from build123d import *
from build123d.topology import SkipClean

# Parameters (mm, degrees)
SKETCH_1_W          = 15
SKETCH_1_H          = 32.4
EXTRUDE_1_DEPTH     = 2.2
SKETCH_1_3_R        = 6.25
SKETCH_1_3_R_2      = 3
CUT_EXTRUDE_1_DEPTH = 36.771497033
SKETCH_2_W          = 15
SKETCH_2_H          = 32.4
EXTRUDE_2_DEPTH     = 4
SKETCH_3_R          = 0.8
CUT_EXTRUDE_2_DEPTH = 3
SKETCH_4_R          = 1
CUT_EXTRUDE_3_DEPTH = 36.927148509
SKETCH_4_3_R        = 1.5
SKETCH_4_3_R_2      = 1
CUT_EXTRUDE_4_DEPTH = 1.2


with BuildPart() as part:
    # Sketch 1 → Extrude 1 (new body)
    with BuildSketch(Plane(origin=(0, 0, 0), x_dir=(1, 0, 0), z_dir=(0, 1, 0))):
        with Locations((7.5, -16.2)):
            Rectangle(SKETCH_1_W, SKETCH_1_H)
    extrude(amount=EXTRUDE_1_DEPTH)

    # Sketch 1_3 → Cut-Extrude 1 (cut, through all)
    with BuildSketch(Plane(origin=(0, 0, 0), x_dir=(1, 0, 0), z_dir=(0, 1, 0))):
        with Locations((7.5, -21.35)):
            Circle(SKETCH_1_3_R)
        with Locations((7.5, -15.6)):
            Circle(SKETCH_1_3_R_2)
    extrude(amount=CUT_EXTRUDE_1_DEPTH, mode=Mode.SUBTRACT)

    # Sketch 2 → Extrude 2 (add)
    with SkipClean():  # the faces are left unmerged after this step: merging them gives an invalid solid
        with BuildSketch(Plane(origin=(0, 2.2, 0), x_dir=(1, 0, 0), z_dir=(0, 1, 0))):
            with Locations((7.5, -16.2)):
                Rectangle(SKETCH_2_W, SKETCH_2_H)
            with BuildLine():
                Line((1.3, -4.5), (13.7, -4.5))
                Line((13.7, -4.5), (13.7, -20.561013308))
                ThreePointArc((13.7, -20.561013308), (13.75, -21.35), (13.7, -22.138986692))
                Line((13.7, -22.138986692), (13.7, -27.9))
                Line((13.7, -27.9), (1.3, -27.9))
                Line((1.3, -27.9), (1.3, -22.138986692))
                ThreePointArc((1.3, -22.138986692), (1.25, -21.35), (1.3, -20.561013308))
                Line((1.3, -20.561013308), (1.3, -4.5))
            make_face(mode=Mode.SUBTRACT)
        extrude(amount=EXTRUDE_2_DEPTH)

    # Sketch 3 → Cut-Extrude 2 (cut)
    with SkipClean():  # the faces are left unmerged after this step: merging them gives an invalid solid
        with BuildSketch(Plane(origin=(0, 6.2, 0), x_dir=(1, 0, 0), z_dir=(0, 1, 0))):
            with Locations(Location((7.5, -30.3, 0), (0, 0, 180))):
                Circle(SKETCH_3_R)
            with Locations(Location((7.5, -2.1, 0), (0, 0, 180))):
                Circle(SKETCH_3_R)
        extrude(amount=-CUT_EXTRUDE_2_DEPTH, mode=Mode.SUBTRACT)

    # Sketch 4 → Cut-Extrude 3 (cut, through all)
    with SkipClean():  # the faces are left unmerged after this step: merging them gives an invalid solid
        with BuildSketch(Plane(origin=(0, 2.2, 0), x_dir=(1, 0, 0), z_dir=(0, 1, 0))):
            with Locations(Location((11.5, -11.35, 0), (0, 0, 270))):
                Circle(SKETCH_4_R)
            with Locations(Location((3.5, -11.35, 0), (0, 0, 270))):
                Circle(SKETCH_4_R)
        extrude(amount=-CUT_EXTRUDE_3_DEPTH, mode=Mode.SUBTRACT)

    # Sketch 4_3 → Cut-Extrude 4 (cut)
    # profile 1 of 2: a face of its own
    with SkipClean():  # the faces are left unmerged after this step: merging them gives an invalid solid
        with BuildSketch(Plane(origin=(0, 2.2, 0), x_dir=(1, 0, 0), z_dir=(0, 1, 0))):
            with Locations(Location((11.5, -11.35, 0), (0, 0, 270))):
                Circle(SKETCH_4_3_R)
            with Locations(Location((11.5, -11.35, 0), (0, 0, 270))):
                Circle(SKETCH_4_3_R_2, mode=Mode.SUBTRACT)
        # profile 2 of 2: a face of its own
        with BuildSketch(Plane(origin=(0, 2.2, 0), x_dir=(1, 0, 0), z_dir=(0, 1, 0))):
            with Locations(Location((3.5, -11.35, 0), (0, 0, 270))):
                Circle(SKETCH_4_3_R)
            with Locations(Location((3.5, -11.35, 0), (0, 0, 270))):
                Circle(SKETCH_4_3_R_2, mode=Mode.SUBTRACT)
        extrude(amount=-CUT_EXTRUDE_4_DEPTH, mode=Mode.SUBTRACT)


solid = part.part
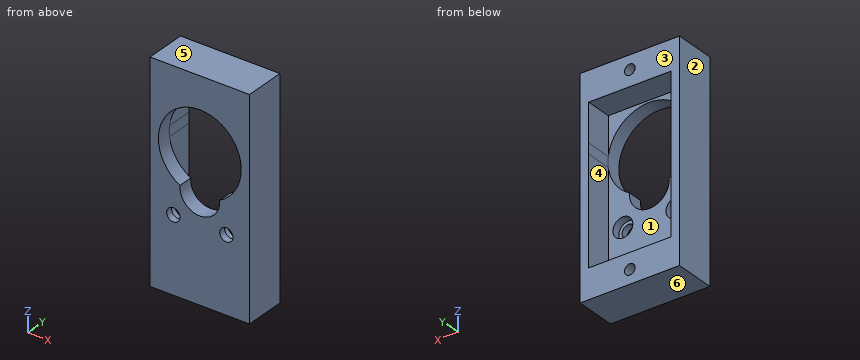
Input: part model. Units: mm. Frame: model coordinates. Face numbers are marked on the shaded views. A direction names the side the tool comes from. Coordinates: 2 decimals unless noted, no trailing zeros. Order: outer loops, then holes, each group sorted by start corner. A loop starts at its lowest first (then second) coordinate and runs counter-clockwise, first axis right, second up. Notation, with made-up numbers: M 88,57.5 L 98,57.5 A20 cw 98,93.5 Z; hole C 28.25,-11.75 d10. An arc over 180 degrees is marked long. Write item = value, one per line. Start each with the question number.
(1) Section A-A on z = 21.35. Output: boundary loops of the cut face in (x, y), and give its area (3 significant figures).
(2) Line query: line 1 along X through (y, z) = (4.75, 14); line 2 along Z through (x, y) = (8.75, 4.75); line 3 along X through (y, z) = (1.1, 15.6). Output: solid intervals per line, ascending. Write a range as [from, to].
(3) Section B-B on y = 4. Output: boundary loops of the cut face in (x, z).
(4) Pull-direction query (Z, two-part tool) for the marked faces 3, 4, 5 and 6; classes: released by +Z, released by -Z, zero draft, split by the parting line, or undercut.
(5) First-contact query: P1, Ø1.3, axis at x = 7.5, z = 30.3, coming from the +Y side; P2, Ø2.5, axis at x = 11, z = 12, coming from the +Y side. Flat tips, straight axial feed; report the tip coordinate or a pass-through.
(6) Reachability of the marked faces 1 and 2 from +Z, -Z, +X, -X, +Y, -Y: full face, straight path, thin tool, end or side. Return the list, or none.
(7) Section D-D on x = 9.25. Output: boundary loops of the cut face in (y, z).
(8) Section C-C on z = 11.35. Output: boundary loops of the cut face in (x, y), and give its area (3 significant figures).
Result set:
q1.outline = M 0,0 L 1.25,0 L 1.25,6.2 L 0,6.2 Z; M 13.75,0 L 15,0 L 15,6.2 L 13.75,6.2 Z
q1.area = 15.5 mm²
q2.line_1 = [0, 1.3], [13.7, 15]
q2.line_2 = [0, 4.5], [27.9, 32.4]
q2.line_3 = [0, 4.5], [10.5, 15]
q3.outline = M 0,0 L 15,0 L 15,32.4 L 0,32.4 Z; hole M 1.3,4.5 L 13.7,4.5 L 13.7,20.56 A6.25 ccw 13.7,22.14 L 13.7,27.9 L 1.3,27.9 L 1.3,22.14 A6.25 ccw 1.3,20.56 Z; hole C 7.5,2.1 d1.6; hole C 7.5,30.3 d1.6
q4.face_3 = zero draft
q4.face_4 = undercut
q4.face_5 = released by +Z
q4.face_6 = released by -Z
q5.P1 = 3.2
q5.P2 = 2.2
q6.face_1 = +Y
q6.face_2 = +Z, -Z, -X, +Y, -Y
q7.outline = M 0,0 L 6.2,0 L 6.2,4.5 L 2.2,4.5 L 2.2,13.16 L 0,13.16 Z; M 0,27.35 L 2.2,27.35 L 2.2,27.9 L 6.2,27.9 L 6.2,32.4 L 0,32.4 Z
q8.outline = M 0,0 L 2.5,0 L 2.5,1 L 2,1 L 2,2.2 L 1.3,2.2 L 1.3,6.2 L 0,6.2 Z; M 4.5,0 L 10.5,0 L 10.5,1 L 10,1 L 10,2.2 L 5,2.2 L 5,1 L 4.5,1 Z; M 12.5,0 L 15,0 L 15,6.2 L 13.7,6.2 L 13.7,2.2 L 13,2.2 L 13,1 L 12.5,1 Z
q8.area = 32.2 mm²
